from build123d import *

# Parameters (mm, degrees)
F1_DEPTH    = 10
F2_T        = 2
F2_T3_DEPTH = 14
F3_R        = 1
F4_DEPTH    = 100


# Not quite as in the source:
# - a shell that OpenCascade refuses in one call is made with other operations: the cavity is built on its own and cut out


with BuildPart() as f1:
    # F0 (on Top) → F1 (new body)
    with BuildSketch(Plane.XY):
        Polygon((-50, 0), (-25, 0), (-37.5, 21.6506350946), align=None)
        Polygon((-12.5, 21.6506350946), (-25, 0), (0, 0), align=None)
        Polygon((12.5, 21.6506350946), (0, 0), (25, 0), align=None)
        Polygon((37.5, 21.6506350946), (25, 0), (50, 0), align=None)
        Polygon((62.5, 21.6506350946), (50, 0), (75, 0), align=None)
        Polygon((0, 0), (-25, 0), (-50, 0), (-50, -1), (75, -1), (75, 0), (50, 0), (25, 0), align=None)
    extrude(amount=F1_DEPTH)

    # F2: shell of thickness 2, made by hand


with BuildPart() as f2_core1:
    # F2_t2: copy of F1
    add(f1.part)

    # the walls: a layer under each face that stays
    f2_faces = [f2_core1.faces().sort_by_distance(p)[0] for p in [
        (-31.25, 10.8253175473, 5),
        (-43.75, 10.8253175473, 5),
        (-50, -0.5, 5),
        (12.5, -1, 5),
        (75, -0.5, 5),
        (68.75, 10.8253175473, 5),
        (56.25, 10.8253175473, 5),
        (43.75, 10.8253175473, 5),
        (31.25, 10.8253175473, 5),
        (18.75, 10.8253175473, 5),
        (6.25, 10.8253175473, 5),
        (-6.25, 10.8253175473, 5),
        (-18.75, 10.8253175473, 5),
        (12.5, 10.3253175473, 0),
        (12.5, 10.3253175473, 10),
    ]]
    thicken(f2_faces, amount=-F2_T, mode=Mode.SUBTRACT)

    # F2_s4 → F2_t3 (cut)
    with BuildSketch(Plane.XY.offset(-2)):
        Polygon((-25, 0.02), (-26.7320508076, -1), (-25, -4), (-23.2679491924, -1), align=None)
        Polygon((50, 0.02), (51.7320508076, -1), (50, -4), (48.2679491924, -1), align=None)
        Polygon((25, 0.02), (26.7320508076, -1), (25, -4), (23.2679491924, -1), align=None)
        Polygon((0, 0.02), (1.7320508076, -1), (0, -4), (-1.7320508076, -1), align=None)
    extrude(amount=F2_T3_DEPTH, mode=Mode.SUBTRACT)


with BuildPart() as f1_1:
    add(f1.part)

    # what is left inside the walls is the cavity
    f2_cavity = [f2_core1.part.solids().sort_by_distance(p)[0] for p in [
        (-37.5, 6.550212, 2.02),
        (-12.5, 6.550212, 2.02),
        (12.5, 6.550212, 2.02),
        (37.5, 6.550212, 2.02),
        (62.5, 6.550212, 2.02),
    ]]
    add(f2_cavity, mode=Mode.SUBTRACT)

    # F3 (on Right) → F4 (cut, symmetric)
    with BuildSketch(Plane.YZ):
        with Locations((17.6506350946, 5)):
            Circle(F3_R)
    extrude(amount=F4_DEPTH, both=True, mode=Mode.SUBTRACT)


solid = f1_1.part
The listing builds one solid part. Answer for the finished solid, in the listing's coordinates (mm). A direction names the side the tool comes from. Coordinates: 2 decimals unless noted, no trailing zeros. Order: outer loops, then holes, each group sorted by start corner. A loop starts at its lowest first (then second) coordinate and runs counter-clockwise, first axis right, second up.
Q1. A cutting plane is placed at A-A, the plane y = 8.5. State how many separate pieces and enclosed holes the cut face has, and give its area (3 significant figures).
Q2. A cutting plane is placed at B-B, the plane x = -30. Write down the section's boundary in (y, z).
Q3. Consider line 1 (Y direction, x = 63.8, z = 5); line 2 (Z direction, x = -19, y = 6); line 3 (Y direction, x = 38.9, z = 5). Determine where each line is inside the solid, lowest interval first.
Q4. Which of the six approach directions +Z, -Z, +X, -X, +Y, -Y give full straight-line access (tool end or side, diameter ignored) to faces 4 (the face through (12.54, 18.11, 4.11)), 5 (the face through (-6.16, 10.67, 4.93)), 6 (the face through (7.76, 9.44, 4.96))?
Q5. Given P1, Ø2.5, axis at y = 17.65, z = 5, coming from the -X side; P2, Ø6, axis at y = 19, z = 9, coming from the -X side; P3, Ø3, axis at x = 66, z = 4.5, coming from the +Y side; P4, Ø12, axis at x = 21, y = 8, coming from the -Z side, each flat-ended and moving along its own axis, determine where each tip first touches the part or whether it passes through.
Q6. For a pull along X with two mould halves and no side action, classify faces 1 (the face through (6.34, 10.98, 4.93)), 2 (the face through (12, 5, 0)), 3 (the face through (62, 1, 5)) as pulls with the +X half, pulls with the -X half, needs draft (parallel to the pull), parting line crosses it, or undercut.
Answers follow:
1. separate pieces: 5
1. enclosed holes: 5
1. area: 442 mm2
2. outline: (-1, 0) - (8.66, 0) - (8.66, 10) - (-1, 10) - close; hole (1, 2) - (4.66, 2) - (4.66, 8) - (1, 8) - close
3. line 1: y = -1 to 1, 15.4 to 16.65, 18.65 to 19.4
3. line 2: z = 0 to 2, 8 to 10
3. line 3: y = -1 to 1, 15.23 to 16.65, 18.65 to 19.23
4. face 4: +X, -X
4. face 5: +Z, -Z, +Y
4. face 6: none
5. P1: stops at x = -40.53
5. P2: stops at x = -40.76
5. P3: stops at y = 18.09
5. P4: stops at z = 0
6. face 1: undercut
6. face 2: needs draft
6. face 3: undercut
